Model file for the job. Use its own axes, mm. Face numbers are marked on the shaded views. Round coordinates to 2 decimals unless told otherwise and drop trailing zeros. Order: outer loops, then holes, each group sorted by start corner. A loop starts at its lowest first (then second) coordinate and runs counter-clockwise, first axis right, second up. Notation, with made-up numbers: (88, 15.25) -> (129, 15.25) arc R24 cw to (129, 27.25) -> close; hole circle Ø10 at (6, 46.5). An arc over 180 degrees is marked (long way). Answer as CSV lines item,"result".
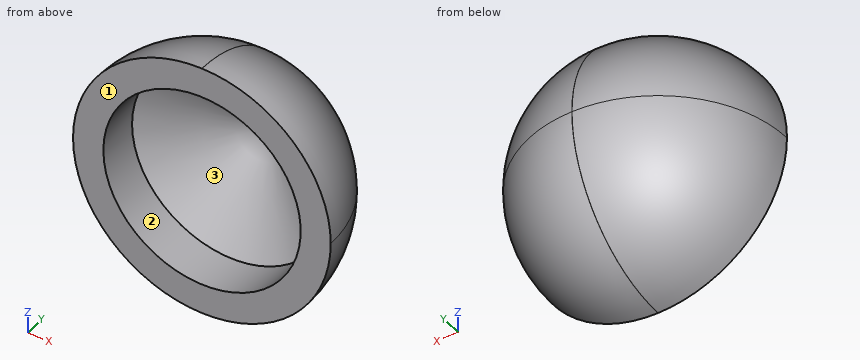
```python
from build123d import *

# Parameters (mm, degrees)
F0_W     = 76.2886069715
F0_H     = 38.1443030201
F1_DEPTH = 76.2
F2_R     = 38.09999
F4_R     = 38.09999
F5_D     = 58.42
F5_DEPTH = 12.7
F5_TIP   = 17.5511386818


# Not quite as in the source:
# - a fillet or chamfer is up to 0.001 mm smaller than in the source, because OpenCascade refuses the exact size


with BuildPart() as f1:
    # F0 (on Top) → F1 (new body)
    with BuildSketch(Plane.XY):
        with Locations((-1.9769910723, 14.3041138072)):
            Rectangle(F0_W, F0_H)
    extrude(amount=F1_DEPTH)

    # F2 (radius 38.1 in the source; OpenCascade refuses exactly that, so slightly less here)
    f2_edges = [f1.edges().sort_by_distance(p)[0] for p in [
        (-40.121295, 14.304114, 76.2),
        (-40.121295, 14.304114, 0),
        (36.167312, 14.304114, 0),
        (36.167312, 14.304114, 76.2),
    ]]
    fillet(f2_edges, radius=F2_R)

    # F4 (radius 38.1 in the source; OpenCascade refuses exactly that, so slightly less here)
    f4_edges = [f1.edges().sort_by_distance(p)[0] for p in [
        (-28.962066, 33.376265, 11.159229),
        (25.008084, 33.376265, 11.159229),
    ]]
    fillet(f4_edges, radius=F4_R)

    # F5
    with Locations(Plane.XZ.offset(4.7680377029)):
        with Locations((-1.9326875865, 38.1)):
            Hole(F5_D / 2, depth=F5_DEPTH)
            with Locations((0, 0, -(F5_DEPTH + F5_TIP / 2))):  # 118° drill point
                Cone(0, F5_D / 2, F5_TIP, mode=Mode.SUBTRACT)


solid = f1.part
```
Q1. Mould opens along X. For the marked faces 1, 2 and 3 say: +X half, -X half, draft (parallel to the pull), parting line (faces both ways), or undercut.
Checks:
face 1,"draft"
face 2,"undercut"
face 3,"undercut"
Q2. Wall check: L1, parallel to X at y = 19.5, z = 35.5; L2, parallel to Z at x = 8, y = 8; L3, parallel to X at y = 4, z = 38 (3 decimals). Give the ranges that are in metal, low to high. Write a range as [from, to].
Checks:
L1,"[-31.31, -11.54], [7.68, 27.36]"
L2,"[3.59, 10.75], [65.45, 72.61]"
L3,"[-39.109, -31.143], [27.277, 35.155]"
Q3. Flat gauge pins, fed straight in: pin 1 (1 mm diameter, centred on x = 6.5, y = 12.5, fed in from +Z); pin 2 (1.5 mm diameter, centred on y = 24.5, z = 22, fed in from +X); pin 3 (2 mm diameter, centred on y = 16.5, z = 10, fed in from -X); pin 4 (6 mm diameter, centred on y = 29, z = 14, fed in from -X). Where does each tip first touch, or does it go through?
Checks:
pin 1,"z = 71.31"
pin 2,"x = 17.76"
pin 3,"x = -18.78"
pin 4,"through"
Q4. Saw through at C-C (z = 6.5). Write the cut outline in (x, y).
Checks:
outline,"(-23.31, -4.77) -> (19.35, -4.77) -> (19.35, -4.72) arc R21.28 ccw to (-1.93, 16.56) -> (-2.02, 16.56) arc R21.28 ccw to (-23.31, -4.72) -> close"
